Autodesk Inventor part; units mm, degrees
ref_plane "YZ Plane" through (0, 0, 0) normal (1, 0, 0) x (0, 1, 0)
ref_plane "XZ Plane" through (0, 0, 0) normal (0, 1, 0) x (-1, 0, 0)
ref_plane "XY Plane" through (0, 0, 0) normal (0, 0, 1) x (1, 0, 0)
sketch "Boceto1" plane through (0, 0, 0) normal (0, 1, 0) x (-1, 0, 0)
  line L0 (0, 145) -> (24.25, 145)
  line L1 (145, 24.25) -> (145, -24.25)
  line L2 (145, 24.25) -> (24.25, 145)
  line L3 (24.25, -145) -> (145, -24.25)
  line L4 (24.25, -145) -> (0, -145)
  circle A0 centre (29.25, -122) radius 2
  circle A1 centre (122, -29.25) radius 2
  circle A2 centre (122, 29.25) radius 2
  circle A3 centre (29.25, 122) radius 2
  line L5 (0, -145) -> (0, 145)
  point P0 (0, 0)
  dimension "d13" = 4
  dimension "d16" = 4
  dimension "d18" = 4
  dimension "d20" = 4
extrude "Extrusión1" add sketch "Boceto1" along normal blind 3
sketch "Boceto5" plane through (0, 3, 0) normal (0, 1, 0) x (1, 0, 0)
  line L0 (-142, 9) -> (-130, 9)
  line L1 (-130, 9) -> (-130, -9)
  line L2 (-130, -9) -> (-142, -9)
  line L3 (-9, -130) -> (-9, -142)
  line L4 (-9, 130) -> (-9, 142)
  line L5 (-142, 9) -> (-142, -9)
  line L6 (-9, -130) -> (0, -130)
  line L7 (-9, -142) -> (0, -142)
  line L8 (0, -130) -> (0, -142)
  line L9 (0, -145) -> (0, 145)
  line L10 (-9, 142) -> (0, 142)
  line L11 (0, 130) -> (0, 142)
  line L12 (-9, 130) -> (0, 130)
extrude "Extrusión5" cut sketch "Boceto5" against normal blind 3
sketch "Boceto8" plane through (0, 3, 0) normal (0, 1, 0) x (1, 0, 0)
  line L0 (0, 24.25) -> (-24.25, 24.25)
  line L1 (0, -24.25) -> (0, 24.25)
  line L2 (-24.25, 24.25) -> (-24.25, -24.25)
  line L3 (-24.25, -24.25) -> (0, -24.25)
extrude "Extrusión8" cut sketch "Boceto8" against normal blind 3
properties part number "_3DPrint"
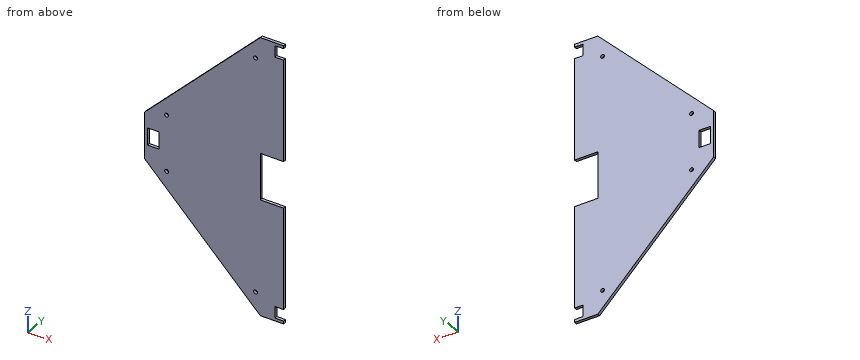
Build history of the part. All positions in model axes, mm. Coordinates: 2 decimals unless noted, no trailing zeros. Write each loop counter-clockwise with the first axis right and the second up, starting at its lowest first coordinate (ties: lowest second). Pieces come first, ordered by that corner, then holes.
(1) Drill centre lines: line 1 (X direction, y = 0.65, z = -1); line 2 (Z direction, x = -122, y = 2.1); line 3 (Z direction, x = -29.25, y = 2.4). Where is each one in solid material? Low to high.
(2) Cut at B-B on x = -69.5. List the corners of the cut face in (y, z).
(3) Pin check, flat tips, straight feed: pin 1 Ø0.9 at (y, z) = (1, 137) entering from +X; pin 2 Ø3.5 at (x, z) = (-29.25, 122) entering from -Y; pin 3 Ø0.9 at (y, z) = (2, 2) entering from +X; pin 4 Ø1 at (y, z) = (2, 46.5) entering from -X. Stop position of each tip, or through.
(4) Cut at C-C on z = -65. List the corners of the cut face in (x, y), and give its area (3 significant figures).
(5) Cut at A-A on y = 2.35. List the corners of the cut face in (x, z), and give its area (3 significant figures).
Working result:
1. line 1: x = -145 to -142, -130 to -24.25
1. line 2: z = -47.25 to -31.25, -27.25 to 27.25, 31.25 to 47.25
1. line 3: z = -140 to -124, -120 to 120, 124 to 140
2. outline: (0, -99.75) - (3, -99.75) - (3, 99.75) - (0, 99.75) - close
3. pin 1: stops at x = -9
3. pin 2: passes through
3. pin 3: stops at x = -24.25
3. pin 4: stops at x = -123.25
4. outline: (-104.25, 0) - (0, 0) - (0, 3) - (-104.25, 3) - close
4. area: 313 mm2
5. outline: (-145, -24.25) - (-24.25, -145) - (0, -145) - (0, -142) - (-9, -142) - (-9, -130) - (0, -130) - (0, -24.25) - (-24.25, -24.25) - (-24.25, 24.25) - (0, 24.25) - (0, 130) - (-9, 130) - (-9, 142) - (0, 142) - (0, 145) - (-24.25, 145) - (-145, 24.25) - close; hole (-142, -9) - (-130, -9) - (-130, 9) - (-142, 9) - close; hole circle Ø4 at (-122, -29.25); hole circle Ø4 at (-122, 29.25); hole circle Ø4 at (-29.25, -122); hole circle Ø4 at (-29.25, 122)
5. area: 25,800 mm2
